Source: three-view drawing plus pictorial views. Frame: mm from the lowest corner of the part. Give positions to 0.01 mm unless a question says otherwise; leave off trailing zeros. Loops run counter-clockwise (first coordinate to the right, second up) from the corner with the lowest first, then second, coordinate; pieces in that order, holes last. Notation, with made-up numbers: M 50,50 L 69,50 A18 ccw 69,62 Z; hole C 6.5,-13 d1. An arc over 180 degrees is marked long. Answer as a JSON object with one key per item and string values. Group by question number.
1) Section query C-C on z = 19. Return loops of the section in (x, y).
2) Ray query, L1, parallel to Y at x = 22.6, z = 8; L2, parallel to X at y = 22, z = 21; L3, parallel to Y at x = 23, z = 7. Return the intervals inside material, ascending.
3) Draft query along Y for the marked faces 1, 2 and 3. Return one class per face: +Y half, -Y half, draft (parallel to the pull), parting line (faces both ways), or undercut.
4) Section query D-D on x = 22.6. Return loops of the section in (y, z).
5) Section query A-A on y = 75. Return loops of the section in (x, z).
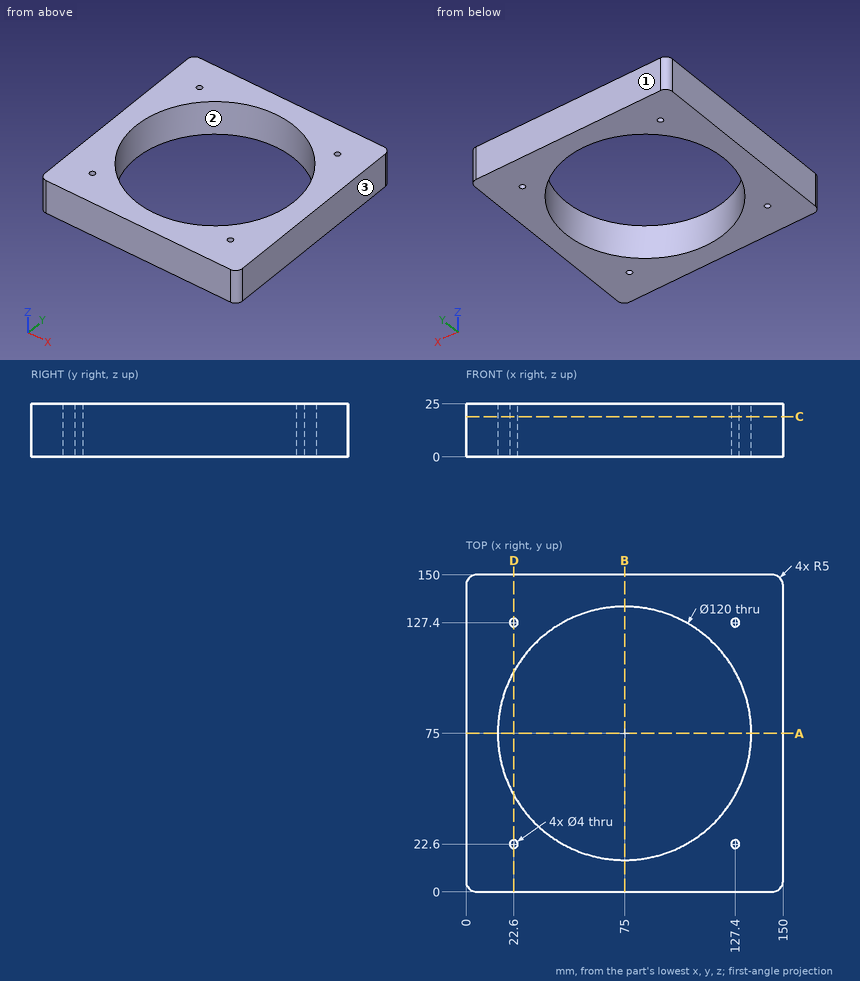
Output:
{
 "1": {"outline": "M 0,5 A5 ccw 5,0 L 145,0 A5 ccw 150,5 L 150,145 A5 ccw 145,150 L 5,150 A5 ccw 0,145 Z; hole C 75,75 d120; hole C 22.6,22.6 d4; hole C 22.6,127.4 d4; hole C 127.4,22.6 d4; hole C 127.4,127.4 d4"},
 "2": {"L1": "y = 0 to 20.6, 24.6 to 45.77, 104.23 to 125.4, 129.4 to 150", "L2": "x = 0 to 20.69, 24.51 to 46.88, 103.12 to 125.49, 129.31 to 150", "L3": "y = 0 to 20.64, 24.56 to 45.07, 104.93 to 125.44, 129.36 to 150"},
 "3": {"face 1": "+Y half", "face 2": "undercut", "face 3": "draft"},
 "4": {"outline": "M 0,0 L 20.6,0 L 20.6,25 L 0,25 Z; M 24.6,0 L 45.77,0 L 45.77,25 L 24.6,25 Z; M 104.23,0 L 125.4,0 L 125.4,25 L 104.23,25 Z; M 129.4,0 L 150,0 L 150,25 L 129.4,25 Z"},
 "5": {"outline": "M 0,0 L 15,0 L 15,25 L 0,25 Z; M 135,0 L 150,0 L 150,25 L 135,25 Z"}
}
